Check sheet for the modelled part. Datum: model origin and axes. Units: mm. A direction names the side the tool comes from. Give positions to 0.01 mm unless a question says otherwise; leave off trailing zeros. Order: outer loops, then holes, each group sorted by start corner. A loop starts at its lowest first (then second) coordinate and runs counter-clockwise, first axis right, second up.
from build123d import *
from OCP.BRepFilletAPI import BRepFilletAPI_MakeChamfer

# Parameters (mm, degrees)
SKETCH_1_W              = 12
SKETCH_1_H              = 46
EXTRUDE_1_DEPTH         = 57
SKETCH_2_W              = 20
SKETCH_2_H              = 46.080872769
CUT_EXTRUDE_1_DEPTH     = 60
SKETCH_3_W              = 12
SKETCH_3_H              = 57
EXTRUDE_2_DEPTH         = 5
SKETCH_4_W              = 12
SKETCH_4_H              = 56
EXTRUDE_3_DEPTH         = 40
SKETCH_5_W              = 12
SKETCH_5_H              = 7
EXTRUDE_4_DEPTH         = 12
M4_A_1_D                = 4.5
M4_A_1_CBORE_D          = 10.705
M4_A_1_CBORE_DEPTH      = 2.8
SKETCH_8_W              = 15
SKETCH_8_H              = 56
EXTRUDE_5_DEPTH         = 3
SKETCH_9_W              = 6
SKETCH_9_H              = 40
CUT_EXTRUDE_2_DEPTH     = 6
CHAMFER_1_SIZE          = 8
CHAMFER_1_SIZE_2        = 5.601660306
SKETCH_10_W             = 6
SKETCH_10_H             = 39.2
EXTRUDE_6_DEPTH         = 9
CUT_EXTRUDE_START       = -4
CUT_EXTRUDE_3_OUTLINE_W = 3
CUT_EXTRUDE_3_OUTLINE_H = 0.4
CUT_EXTRUDE_3_DEPTH     = 5
CHAMFER_2_SIZE          = 1
CHAMFER_3_SIZE          = 2
CHAMFER_3_SIZE2         = 1.400415076
SKETCH_12_W             = 45
SKETCH_12_H             = 20.5
CUT_EXTRUDE_4_DEPTH     = 4
SKETCH_14_W             = 7
SKETCH_14_H             = 80
EXTRUDE_7_DEPTH         = 10
CUT_EXTRUDE_5_DEPTH     = 102.271911209
SKETCH_16_W             = 3
SKETCH_16_H             = 56
EXTRUDE_8_DEPTH         = 12
CHAMFER_5_SIZE          = 5
CUT_EXTRUDE_START_2     = -42.060641
SKETCH_17_W             = 3
SKETCH_17_H             = 56
CUT_EXTRUDE_6_DEPTH     = 42.060641
CHAMFER_4_SIZE          = 1
FILLET_1_R              = 12
SKETCH_22_W             = 3
SKETCH_22_H             = 80
EXTRUDE_11_DEPTH        = 0.8
SKETCH_24_W             = 9
SKETCH_24_H             = 2
EXTRUDE_13_DEPTH        = 1


with BuildPart() as part:
    # Sketch 1 → Extrude 1 (new body)
    with BuildSketch(Plane.XY):
        Rectangle(SKETCH_1_W, SKETCH_1_H)
    extrude(amount=EXTRUDE_1_DEPTH)

    # Sketch 2 → Cut-Extrude 1 (cut)
    with BuildSketch(Plane(origin=(6, 0, 0), x_dir=(0, 0, -1), z_dir=(1, 0, 0))):
        with Locations((-30, 0.040436385)):
            Rectangle(SKETCH_2_W, SKETCH_2_H)
    extrude(amount=-CUT_EXTRUDE_1_DEPTH, mode=Mode.SUBTRACT)


with BuildPart() as cut_extrude_1_piece_1:
    # of the separate pieces the step leaves, piece 1, a body of its own (cut_extrude_1_pieces)
    add(part.part.solids().sort_by_distance((-6, 23, 0))[0])



with BuildPart() as cut_extrude_1_piece_2:
    # of the separate pieces the step leaves, piece 2, a body of its own (cut_extrude_1_pieces)
    add(part.part.solids().sort_by_distance((6, 23, 40))[0])


with BuildPart() as cut_extrude_1_piece_1_1:
    add(cut_extrude_1_piece_1.part)

    add(cut_extrude_1_piece_2.part)  # Extrude 2 merges Cut-Extrude 1 piece 2
    # Sketch 3 → Extrude 2 (add)
    with BuildSketch(Plane.XZ.offset(23)):
        with Locations((0, 28.5)):
            Rectangle(SKETCH_3_W, SKETCH_3_H)
    extrude_2 = extrude(amount=EXTRUDE_2_DEPTH)

    # Mirror 1: Extrude 2 across plane
    add(extrude_2.mirror(Plane.ZX))

    # Sketch 4 → Extrude 3 (add)
    with BuildSketch(Plane(origin=(0, 0, 0), x_dir=(-1, 0, 0), z_dir=(0, 0, -1))):
        Rectangle(SKETCH_4_W, SKETCH_4_H)
    extrude(amount=EXTRUDE_3_DEPTH)

    # Sketch 5 → Extrude 4 (add)
    with BuildSketch(Plane.XZ.offset(28)):
        with Locations((0, -36.5)):
            Rectangle(SKETCH_5_W, SKETCH_5_H)
    extrude_4 = extrude(amount=EXTRUDE_4_DEPTH)

    # Mirror 2: Extrude 4 across plane
    add(extrude_4.mirror(Plane.ZX))

    # M4 _ _ _ _ _A _1 (through all)
    with Locations(Plane.XY.offset(-33)):
        with Locations((0, -34), (0, 34)):
            CounterBoreHole(M4_A_1_D / 2, M4_A_1_CBORE_D / 2, M4_A_1_CBORE_DEPTH)

    # Sketch 8 → Extrude 5 (add)
    with BuildSketch(Plane.XY.offset(57)):
        with Locations((-1.5, 0)):
            Rectangle(SKETCH_8_W, SKETCH_8_H)
    extrude(amount=EXTRUDE_5_DEPTH)

    # Sketch 9 → Cut-Extrude 2 (cut)
    with BuildSketch(Plane.XY.offset(60)):
        with Locations((3, 0)):
            Rectangle(SKETCH_9_W, SKETCH_9_H)
    extrude(amount=-CUT_EXTRUDE_2_DEPTH, mode=Mode.SUBTRACT)

    # Chamfer 1
    chamfer_1_edges_1 = [cut_extrude_1_piece_1_1.edges().sort_by_distance(p)[0] for p in [
        (0, 0, 60),
    ]]
    chamfer_1_side_1 = [cut_extrude_1_piece_1_1.faces().sort_by_distance(p)[0] for p in [
        (-0.112033206, 0, 60),
    ]]
    chamfer_1_edges_2 = [cut_extrude_1_piece_1_1.edges().sort_by_distance(p)[0] for p in [
        (3, 20, 60),
    ]]
    chamfer_1_side_2 = [cut_extrude_1_piece_1_1.faces().sort_by_distance(p)[0] for p in [
        (3, 20.112033206, 60),
    ]]
    chamfer_1_edges_3 = [cut_extrude_1_piece_1_1.edges().sort_by_distance(p)[0] for p in [
        (3, -20, 60),
    ]]
    chamfer_1_side_3 = [cut_extrude_1_piece_1_1.faces().sort_by_distance(p)[0] for p in [
        (3, -20.112033206, 60),
    ]]
    chamfer_1 = BRepFilletAPI_MakeChamfer(cut_extrude_1_piece_1_1.part.solid().wrapped)
    for e in chamfer_1_edges_1:
        chamfer_1.Add(CHAMFER_1_SIZE - 0.0001, CHAMFER_1_SIZE_2 - 0.0001, e.wrapped, chamfer_1_side_1[0].wrapped)
    for e in chamfer_1_edges_2:
        chamfer_1.Add(CHAMFER_1_SIZE - 0.0001, CHAMFER_1_SIZE_2 - 0.0001, e.wrapped, chamfer_1_side_2[0].wrapped)
    for e in chamfer_1_edges_3:
        chamfer_1.Add(CHAMFER_1_SIZE - 0.0001, CHAMFER_1_SIZE_2 - 0.0001, e.wrapped, chamfer_1_side_3[0].wrapped)
    add(Compound.cast(chamfer_1.Shape()), mode=Mode.REPLACE)  # a hair under: the kernel refuses the full size

    # Sketch 10 → Extrude 6 (add)
    with BuildSketch(Plane(origin=(0, 0, -40), x_dir=(-1, 0, 0), z_dir=(0, 0, -1))):
        with Locations((-3, 0)):
            Rectangle(SKETCH_10_W, SKETCH_10_H)
    extrude(amount=EXTRUDE_6_DEPTH)

    # Cut-Extrude 3: read off the stored shape, not the designer's step
    # Cut-Extrude 3 outline → Cut-Extrude 3 (cut)
    with BuildSketch(Plane.XY.offset(60).offset(CUT_EXTRUDE_START)):
        with Locations((-7.5, 27.8)):
            Rectangle(CUT_EXTRUDE_3_OUTLINE_W, CUT_EXTRUDE_3_OUTLINE_H)
        with Locations((-7.5, -27.8)):
            Rectangle(CUT_EXTRUDE_3_OUTLINE_W, CUT_EXTRUDE_3_OUTLINE_H)
    extrude(amount=CUT_EXTRUDE_3_DEPTH, mode=Mode.SUBTRACT)

    # Chamfer 2
    chamfer_2_edges = [cut_extrude_1_piece_1_1.edges().sort_by_distance(p)[0] for p in [
        (-7.5, -27.6, 57),
        (-7.5, 27.6, 57),
    ]]
    chamfer(chamfer_2_edges, length=CHAMFER_2_SIZE)

    # Chamfer 3: one chamfer whose edges measure the first distance from different faces: ONE call of the kernel's chamfer builder (chamfer() names one face for all edges)
    chamfer_3_edges_1 = [cut_extrude_1_piece_1_1.edges().sort_by_distance(p)[0] for p in [
        (6, 0, -49),
    ]]
    chamfer_3_side_1 = [cut_extrude_1_piece_1_1.faces().sort_by_distance(p)[0] for p in [
        (6, 0, -1.976539193),
    ]]
    chamfer_3_edges_2 = [cut_extrude_1_piece_1_1.edges().sort_by_distance(p)[0] for p in [
        (3, -19.6, -49),
    ]]
    chamfer_3_side_2 = [cut_extrude_1_piece_1_1.faces().sort_by_distance(p)[0] for p in [
        (3, -19.6, -44.5),
    ]]
    chamfer_3_edges_3 = [cut_extrude_1_piece_1_1.edges().sort_by_distance(p)[0] for p in [
        (0, 0, -49),
    ]]
    chamfer_3_side_3 = [cut_extrude_1_piece_1_1.faces().sort_by_distance(p)[0] for p in [
        (0, 0, -44.5),
    ]]
    chamfer_3_edges_4 = [cut_extrude_1_piece_1_1.edges().sort_by_distance(p)[0] for p in [
        (3, 19.6, -49),
    ]]
    chamfer_3_side_4 = [cut_extrude_1_piece_1_1.faces().sort_by_distance(p)[0] for p in [
        (3, 19.6, -44.5),
    ]]
    chamfer_3 = BRepFilletAPI_MakeChamfer(cut_extrude_1_piece_1_1.part.solid().wrapped)
    for e in chamfer_3_edges_1:
        chamfer_3.Add(CHAMFER_3_SIZE, CHAMFER_3_SIZE2, e.wrapped, chamfer_3_side_1[0].wrapped)  # the first distance lies on this face
    for e in chamfer_3_edges_2:
        chamfer_3.Add(CHAMFER_3_SIZE, CHAMFER_3_SIZE2, e.wrapped, chamfer_3_side_2[0].wrapped)  # the first distance lies on this face
    for e in chamfer_3_edges_3:
        chamfer_3.Add(CHAMFER_3_SIZE, CHAMFER_3_SIZE2, e.wrapped, chamfer_3_side_3[0].wrapped)  # the first distance lies on this face
    for e in chamfer_3_edges_4:
        chamfer_3.Add(CHAMFER_3_SIZE, CHAMFER_3_SIZE2, e.wrapped, chamfer_3_side_4[0].wrapped)  # the first distance lies on this face
    add(Compound.cast(chamfer_3.Shape()), mode=Mode.REPLACE)

    # Sketch 12 → Cut-Extrude 4 (cut)
    with BuildSketch(Plane.ZY.offset(6)):
        with Locations((-7.5, 12.75)):
            Rectangle(SKETCH_12_W, SKETCH_12_H)
        with Locations((-7.5, -12.75)):
            Rectangle(SKETCH_12_W, SKETCH_12_H)
    cut_extrude_4 = extrude(amount=-CUT_EXTRUDE_4_DEPTH, mode=Mode.SUBTRACT)

    # Mirror 3: Cut-Extrude 4 across plane
    add(cut_extrude_4.mirror(Plane.ZY), mode=Mode.SUBTRACT)

    # Sketch 14 → Extrude 7 (add)
    with BuildSketch(Plane(origin=(6, 0, 0), x_dir=(0, 0, -1), z_dir=(1, 0, 0))):
        with Locations((36.5, 0)):
            Rectangle(SKETCH_14_W, SKETCH_14_H)
    extrude(amount=EXTRUDE_7_DEPTH)

    # Sketch 15 → Cut-Extrude 5 (cut, through all)
    with BuildSketch(Plane.XZ.offset(40)):
        with BuildLine():
            Line((6, -33), (16, -33))
            Line((16, -33), (16, -28.353890031))
            add(Edge.make_bspline(
                [(6, -33), (5.579283, -24.005465365), (9.542787604, -28.181394392), (15.145388019, -28.353890031), (16, -28.353890031)],
                knots=[0, 0, 0, 0, 0.752787833, 1, 1, 1, 1], degree=3))
        make_face()
    extrude(amount=-CUT_EXTRUDE_5_DEPTH, mode=Mode.SUBTRACT)

    # Sketch 16 → Extrude 8 (add)
    with BuildSketch(Plane(origin=(6, 0, 0), x_dir=(0, 0, -1), z_dir=(1, 0, 0))):
        with Locations((-16.43935887, 0)):
            Rectangle(SKETCH_16_W, SKETCH_16_H)
    extrude(amount=EXTRUDE_8_DEPTH)

    # Chamfer 5
    chamfer_5_edges = [cut_extrude_1_piece_1_1.edges().sort_by_distance(p)[0] for p in [
        (16, 0, -33),
    ]]
    chamfer(chamfer_5_edges, length=CHAMFER_5_SIZE)

    # Sketch 17 → Cut-Extrude 6 (cut)
    with BuildSketch(Plane.XY.offset(60).offset(CUT_EXTRUDE_START_2)):
        with Locations((4.5, 0)):
            Rectangle(SKETCH_17_W, SKETCH_17_H)
    extrude(amount=CUT_EXTRUDE_6_DEPTH, mode=Mode.SUBTRACT)

    # Chamfer 4
    chamfer_4_edges = [cut_extrude_1_piece_1_1.edges().sort_by_distance(p)[0] for p in [
        (3, -23, 30),
        (3, 23, 30),
        (3, 0, 20),
        (3, 0, 40),
    ]]
    chamfer(chamfer_4_edges, length=CHAMFER_4_SIZE)

    # Fillet 1
    fillet_1_edges = [cut_extrude_1_piece_1_1.edges().sort_by_distance(p)[0] for p in [
        (6, -25.5, 14.93935887),
        (6, 0, 14.93935887),
        (6, 25.5, 14.93935887),
    ]]
    fillet(fillet_1_edges, radius=FILLET_1_R - 0.0001)  # a hair under: the kernel refuses the full size

    # Sketch 22 → Extrude 11 (add)
    with BuildSketch(Plane(origin=(0, 0, -40), x_dir=(-1, 0, 0), z_dir=(0, 0, -1))):
        with Locations((-14.5, 0)):
            Rectangle(SKETCH_22_W, SKETCH_22_H)
    extrude(amount=EXTRUDE_11_DEPTH)

    # Sketch 24 → Extrude 13 (add)
    with BuildSketch(Plane(origin=(0, 28, 0), x_dir=(1, 0, 0), z_dir=(0, 1, 0))):
        with Locations((-1.5, -59)):
            Rectangle(SKETCH_24_W, SKETCH_24_H)
    extrude_13 = extrude(amount=EXTRUDE_13_DEPTH)

    # Mirror 4: Extrude 13 across plane
    add(extrude_13.mirror(Plane.ZX))


solid = cut_extrude_1_piece_1_1.part
1) Section check A-A, the plane y = 34. Record the cut outline in (x, z), then the cut area to 3 significant figures.
Recorded:
outline: (-6, -40) - (-2.25, -40) - (-2.25, -35.8) - (-5.35, -35.8) - (-5.35, -33) - (-6, -33) - close; (2.25, -40) - (13, -40) - (13, -40.8) - (16, -40.8) - (16, -38) - (11, -33) - (5.35, -33) - (5.35, -35.8) - (2.25, -35.8) - close
area: 95.0 mm2
2) Draft check along X on faces 1 (the face through (-1.2, -24.83, 57.78)), 2 (the face through (-6, 1, 11)), 3 (the face through (8, -1, -40)). Enter one of: +X half, -X half, draft (parallel to the pull), parting line (faces both ways), or undercut.
Recorded:
face 1: draft
face 2: -X half
face 3: undercut
3) Set-up check for faces 4 (the face through (1, 0, 54)), 5 (the face through (0, -28, 3)), 6 (the face through (4, -13, -30)): record each of +Z, -Z, +X, -X, +Y, -Y from which the full face is reachable in a straight line by a thin tool's end or side.
Recorded:
face 4: +Z, +X
face 5: +X, -X, -Y
face 6: +X
4) Depth check by flat-ended pin: pin 1 Ø10 at (y, z) = (9, 39.5) entering from -X; pin 2 Ø10 at (y, z) = (-2.5, -10.5) entering from +X; pin 3 Ø0.6 at (x, z) = (-7, 59) entering from -Y. Enter the tip coordinate at first touch or a pass-through.
Recorded:
pin 1: stops at x = -6
pin 2: stops at x = 6
pin 3: stops at y = -27.6
5) Material ranges on L1, parallel to Y at x = 0, z = -38.5; L2, parallel to Y at x = 0, z = -34.45; L3, parallel to Z at x = -5, y = -6.5, recorded low to high.
Recorded:
L1: y = -40 to -36.25, -31.75 to 31.75, 36.25 to 40
L2: y = -40 to -39.35, -28.65 to 28.65, 39.35 to 40
L3: z = -40 to -30, 15 to 20, 40 to 57.9
6) Section check B-B, the plane z = -2. Record the cut outline in (x, y).
Recorded:
outline: (-6, -28) - (6, -28) - (6, -23) - (2, -23) - (2, -2.5) - (6, -2.5) - (6, 2.5) - (2, 2.5) - (2, 23) - (6, 23) - (6, 28) - (-6, 28) - (-6, 23) - (-2, 23) - (-2, 2.5) - (-6, 2.5) - (-6, -2.5) - (-2, -2.5) - (-2, -23) - (-6, -23) - close
